from build123d import *

# Parameters (mm, degrees)
BOSS_EXTRUDE1_DEPTH = 10
SKETCH2_R           = 2
CUT_EXTRUDE1_DEPTH  = 116.971936943
FILLET1_R           = 2


with BuildPart() as part:
    # Sketch1 → Boss-Extrude1 (new body)
    with BuildSketch(Plane(origin=(0, 0, 0), x_dir=(0, 1, 0), z_dir=(0, 0, 1))):
        with BuildLine():
            Line((-36.324229872, 27.68131099), (-51.324229872, 23.662073103))
            Line((-51.324229872, 23.662073103), (-33.907532364, -41.337926897))
            ThreePointArc((-33.907532364, -41.337926897), (-35.409341514, -51.440004773), (-29.149202114, -59.509581147))
            Line((-29.149202114, -59.509581147), (-19.739589339, -103.514798876))
            Line((-19.739589339, -103.514798876), (-9.739589339, -103.514798876))
            Line((-9.739589339, -103.514798876), (-9.739589339, -100.514798876))
            Line((-9.739589339, -100.514798876), (-6.545356821, -20.514798876))
            Line((-6.545356821, -20.514798876), (-12.545356821, -25.337926897))
            Line((-12.545356821, -25.337926897), (-19.535457388, -41.337926897))
            Line((-19.535457388, -41.337926897), (-27.535457388, -34.854054639))
            Line((-27.535457388, -34.854054639), (-36.324229872, 27.68131099))
        make_face()
    extrude(amount=BOSS_EXTRUDE1_DEPTH)

    # Sketch2 → Cut-Extrude1 (cut, through all)
    with BuildSketch(Plane.XY.offset(10)):
        with Locations((-20.833645978, -46.425250386)):
            Circle(SKETCH2_R)
    extrude(amount=-CUT_EXTRUDE1_DEPTH, mode=Mode.SUBTRACT)

    # Fillet1
    fillet1_edges = [part.edges().sort_by_distance(p)[0] for p in [
        (59.509581147, -29.149202114, 5),
        (41.337926897, -33.907532364, 5),
        (-23.662073103, -51.324229872, 5),
        (-27.68131099, -36.324229872, 5),
        (34.854054639, -27.535457388, 5),
        (41.337926897, -19.535457388, 5),
        (25.337926897, -12.545356821, 5),
        (20.514798876, -6.545356821, 5),
    ]]
    fillet(fillet1_edges, radius=FILLET1_R)


solid = part.part
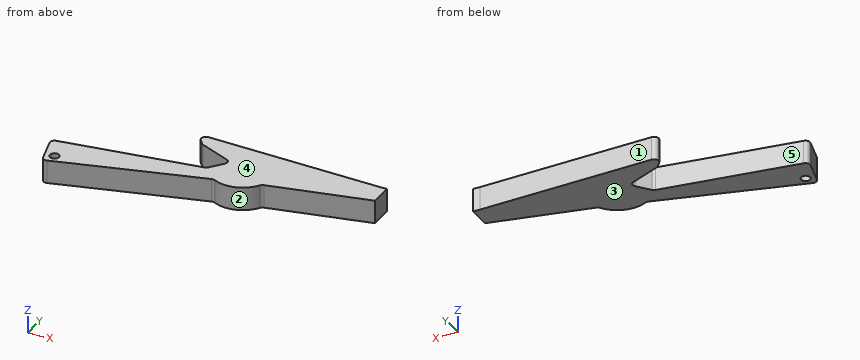
Build history of the part. All positions in model axes, mm. Face numbers are marked on the shaded views. A direction names the side the tool comes from. Give positions to 0.01 mm unless a question says otherwise; leave off trailing zeros. Loops run counter-clockwise (first coordinate to the right, second up) from the corner with the lowest first, then second, coordinate; pieces in that order, holes last. Notation, with made-up numbers: (-31, -20) -> (1, -20) arc R29 ccw to (1, 8) -> close; hole circle Ø9 at (-32, -26.75). An arc over 180 degrees is marked (long way). Answer in a Markdown table with one row per item.
Item 1: Slice it at A-A on z = 7.5. Write the cut outline in (x, y).
Findings below:
| item | result |
|---|---|
| outline | (-27.1, -38.51) -> (-24.18, -49.39) arc R2 ccw to (-21.73, -50.81) -> (40.54, -34.12) arc R2 cw to (42, -34.29) arc R13 ccw to (59.09, -29.84) arc R2 cw to (60.36, -28.97) -> (103.51, -19.74) -> (103.51, -9.74) -> (100.51, -9.74) -> (24.91, -6.72) arc R2 ccw to (23.27, -9.97) -> (25.03, -12.16) arc R2 ccw to (25.79, -12.74) -> (38.93, -18.48) arc R2 cw to (39.68, -21.58) -> (35.35, -26.92) arc R2 cw to (34.07, -27.65) -> (-25.44, -36.01) arc R2 ccw to start; hole circle Ø4 at (-20.83, -46.43) |
Item 2: Slice it at B-B on y = -16.5. Write the cut outline in (x, z), plus the area to 3 significant figures.
Findings below:
| item | result |
|---|---|
| outline | (34.39, 0) -> (103.51, 0) -> (103.51, 10) -> (34.39, 10) -> close |
| area | 691 mm² |
Item 3: Mould opens along X. For the marked faces 1, 2 and 3 say: pulls with the +X half, pulls with the -X half, needs draft (parallel to the pull), parting line crosses it, or undercut.
Findings below:
| item | result |
|---|---|
| face 1 | pulls with the +X half |
| face 2 | undercut |
| face 3 | needs draft |
Item 4: Probe line 1 along Y through (x, z) = (-20.5, 1.25); line 2 along Y through (x, z) = (31, 5.5); line 3 along X through (y, z) = (-17.5, 7.75). List the from-to ranges inside material, lowest first. Write a range as [from, to].
Findings below:
| item | result |
|---|---|
| line 1 | y = [-50.48, -48.4], [-44.45, -35.31] |
| line 2 | y = [-36.68, -28.08], [-15.02, -6.96] |
| line 3 | x = [36.68, 103.51] |
Item 5: Flat gauge pins, fed straight in: P1, Ø3.5, axis at x = 102, z = 5, coming from the +Y side; P2, Ø5, axis at x = -20.83, y = -46.43, coming from the +Z side; P3, Ø4, axis at y = -45.5, z = 3.5, coming from the -X side; P4, Ø1, axis at y = -26, z = 8.5, coming from the -X side. Where does each tip first touch, or does it go through?
Findings below:
| item | result |
|---|---|
| P1 | stops at y = -9.73 |
| P2 | stops at z = 10 |
| P3 | stops at x = -25.76 |
| P4 | stops at x = 35.69 |
Item 6: Slice it at C-C on x = 13. Write the cut outline in (y, z).
Findings below:
| item | result |
|---|---|
| outline | (-41.5, 0) -> (-30.61, 0) -> (-30.61, 10) -> (-41.5, 10) -> close |
Item 7: Tool access for the marked faces 4 and 5: list every direction of +Z, -Z, +X, -X, +Y, -Y with a clear straight run to the whole face (end or side of a thin tool).
Findings below:
| item | result |
|---|---|
| face 4 | +Z, +X, -X, +Y, -Y |
| face 5 | +Z, -Z, -X |
